Work out the finished part from the listing and answer in its coordinate system (mm). Face numbers are marked on the shaded views. A direction names the side the tool comes from. Coordinates: 2 decimals unless noted, no trailing zeros. Order: outer loops, then holes, each group sorted by start corner. A loop starts at its lowest first (then second) coordinate and runs counter-clockwise, first axis right, second up. Notation, with made-up numbers: M -33,74 L -24,74 A13 ccw -24,95 Z; hole C -5,-25.75 d4. An arc over 180 degrees is marked long. Use a Markdown table: item, result.
from build123d import *

# Parameters (mm, degrees)
F0_R     = 6.3
F0_R_2   = 6
F2_DEPTH = 6
F3_R     = 1.5
F4_DEPTH = 8.128
F5_R     = 1.2
F6_DEPTH = 25.4
F7_DEPTH = 4.3


with BuildPart() as f2:
    # F0 (on Top) → F2 (new body)
    with BuildSketch(Plane.XY):
        Circle(F0_R)
        Circle(F0_R_2, mode=Mode.SUBTRACT)
        Circle(F0_R_2)
    extrude(amount=F2_DEPTH)

    # F3 (on face) → F4 (join)
    with BuildSketch(Plane.XY.offset(6)):
        Circle(F3_R)
    extrude(amount=F4_DEPTH)

    # F5 (on face) → F6 (cut)
    with BuildSketch(Plane.XY.offset(14.128)):
        Circle(F5_R)
    extrude(amount=-F6_DEPTH, mode=Mode.SUBTRACT)

    # F0 (on Top) → F7 (cut)
    with BuildSketch(Plane.XY):
        Circle(F0_R_2)
    extrude(amount=F7_DEPTH, mode=Mode.SUBTRACT)


solid = f2.part
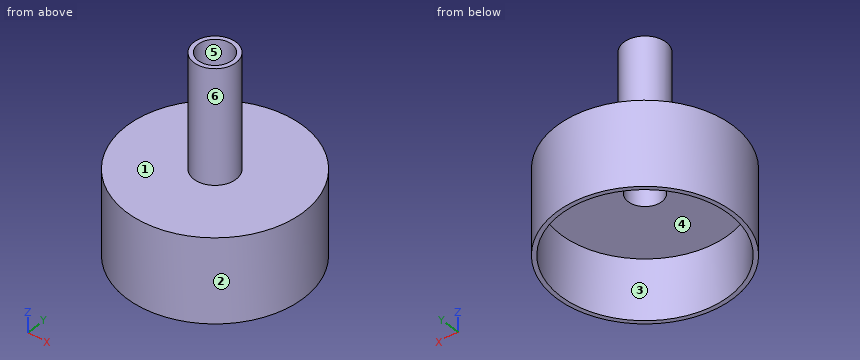
(1) A cutting plane is placed at A-A (x = 0). Determine the outline of the cut face in (y, z).
Conclusion:
| item | result |
|---|---|
| outline | M -6.3,0 L -6,0 L -6,4.3 L -1.2,4.3 L -1.2,14.13 L -1.5,14.13 L -1.5,6 L -6.3,6 Z; M 1.2,4.3 L 6,4.3 L 6,0 L 6.3,0 L 6.3,6 L 1.5,6 L 1.5,14.13 L 1.2,14.13 Z |
(2) A cutting plane is placed at D-D (y = 5.5). Determine the outline of the cut face in (x, z), then the cut area to 3 significant figures.
Conclusion:
| item | result |
|---|---|
| outline | M -3.07,0 L -2.4,0 L -2.4,4.3 L 2.4,4.3 L 2.4,0 L 3.07,0 L 3.07,6 L -3.07,6 Z |
| area | 16.2 mm2 |
(3) Which of the six approach directions +Z, -Z, +X, -X, +Y, -Y give full straight-line access (tool end or side, diameter ignored) to the marked faces 4, 5 and 6?
Conclusion:
| item | result |
|---|---|
| face 4 | -Z |
| face 5 | +Z, -Z |
| face 6 | +Z |
(4) Determine the mould class of the marked faces 1, 2 and 3 for opening direction X: pulls with the +X half, pulls with the -X half, needs draft (parallel to the pull), parting line crosses it, or undercut.
Conclusion:
| item | result |
|---|---|
| face 1 | needs draft |
| face 2 | parting line crosses it |
| face 3 | undercut |
(5) Given P1, Ø4, axis at y = 5, z = 3.5, coming from the -X side; P2, Ø1, axis at x = 3, y = 3, coming from the +Z side; P3, Ø1, axis at x = 3.5, y = 2.5, coming from the -Z side, each flat-ended and moving along its own axis, determine where each tip first touches the part or whether it passes through.
Conclusion:
| item | result |
|---|---|
| P1 | x = -5.54 |
| P2 | z = 6 |
| P3 | z = 4.3 |
(6) A cutting plane is placed at C-C (z = 8). Determine the outline of the cut face in (x, y), then the cut area to 3 significant figures.
Conclusion:
| item | result |
|---|---|
| outline | C 0,0 d3; hole C 0,0 d2.4 |
| area | 2.54 mm2 |
(7) A cutting plane is placed at B-B (y = 1). Determine the outline of the cut face in (x, z), then the cut area to 3 significant figures.
Conclusion:
| item | result |
|---|---|
| outline | M -6.22,0 L -5.92,0 L -5.92,4.3 L -0.66,4.3 L -0.66,14.13 L -1.12,14.13 L -1.12,6 L -6.22,6 Z; M 0.66,4.3 L 5.92,4.3 L 5.92,0 L 6.22,0 L 6.22,6 L 1.12,6 L 1.12,14.13 L 0.66,14.13 Z |
| area | 28.9 mm2 |
(8) Straight lines are drawn through the part: L1, parallel to Y at x = 0, z = 2.15; L2, parallel to Y at x = 0, z = 11.5; L3, parallel to Z at x = 1, y = -6. For each, find the intervals that lie inside material, in ascending order.
Conclusion:
| item | result |
|---|---|
| L1 | -6.3 to -6, 6 to 6.3 |
| L2 | -1.5 to -1.2, 1.2 to 1.5 |
| L3 | 0 to 6 |
